Geometry check sheet. Reference: the model listing, model coordinates, mm. Face numbers are marked on the shaded views. Coordinates: 2 decimals unless noted, no trailing zeros. Loops run counter-clockwise (first coordinate to the right, second up) from the corner with the lowest first, then second, coordinate; pieces in that order, holes last.
from build123d import *

# Parameters (mm, degrees)
F0_W     = 266.7
F0_H     = 152.4
F0_R     = 19.05
F1_DEPTH = 50.8
F2_R     = 6.35


with BuildPart() as f1:
    # F0 (on Front) → F1 (new body)
    with BuildSketch(Plane.XZ):
        Rectangle(F0_W, F0_H)
        with Locations((-63.5, 0)):
            Circle(F0_R, mode=Mode.SUBTRACT)
        with BuildLine():
            ThreePointArc((-19.05, 0), (0, 19.05), (19.05, 0))
            ThreePointArc((19.05, 0), (0, -19.05), (-19.05, 0))
        make_face(mode=Mode.SUBTRACT)
        with BuildLine():
            ThreePointArc((82.55, 0), (63.5, -19.05), (44.45, 0))
            ThreePointArc((44.45, 0), (63.5, 19.05), (82.55, 0))
        make_face(mode=Mode.SUBTRACT)
    extrude(amount=F1_DEPTH)

    # F2
    f2_edges = [f1.edges().sort_by_distance(p)[0] for p in [
        (0, -50.8, 76.2),
        (-133.35, -50.8, 0),
        (0, -50.8, -76.2),
        (133.35, -50.8, 0),
    ]]
    fillet(f2_edges, radius=F2_R)


solid = f1.part
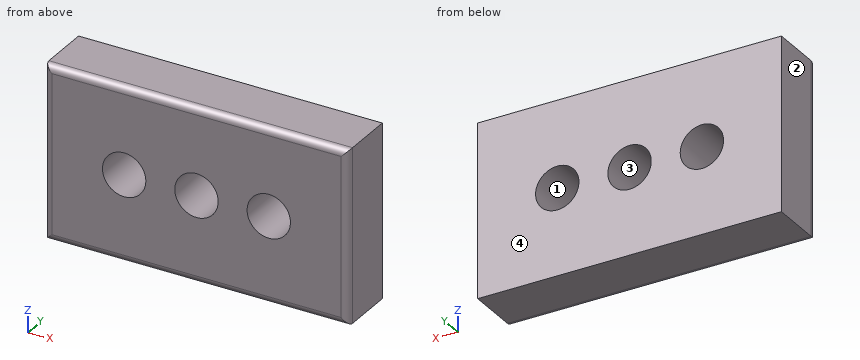
(1) Sectioned sample at D-D on x = -51. Record the cut outline in (y, z).
Findings:
outline: (-50.8, -69.85) arc R6.35 ccw to (-44.45, -76.2) - (0, -76.2) - (0, -14.38) - (-50.8, -14.38) - close; (-50.8, 14.38) - (0, 14.38) - (0, 76.2) - (-44.45, 76.2) arc R6.35 ccw to (-50.8, 69.85) - close
(2) Sectioned sample at A-A on z = 0. Record the cut outline in (x, y), and give its area (3 significant figures).
Findings:
outline: (-133.35, -44.45) arc R6.35 ccw to (-127, -50.8) - (-82.55, -50.8) - (-82.55, 0) - (-133.35, 0) - close; (-44.45, -50.8) - (-19.05, -50.8) - (-19.05, 0) - (-44.45, 0) - close; (19.05, -50.8) - (44.45, -50.8) - (44.45, 0) - (19.05, 0) - close; (82.55, -50.8) - (127, -50.8) arc R6.35 ccw to (133.35, -44.45) - (133.35, 0) - (82.55, 0) - close
area: 7,720 mm2
(3) Draft check along X on the marked faces 1, 2, 3 and 4. Enter one of: +X half, -X half, draft (parallel to the pull), parting line (faces both ways), or undercut.
Findings:
face 1: undercut
face 2: -X half
face 3: undercut
face 4: draft
(4) Sectioned sample at C-C on x = 63.5. Record the cut outline in (y, z), and give its area (3 significant figures).
Findings:
outline: (-50.8, -69.85) arc R6.35 ccw to (-44.45, -76.2) - (0, -76.2) - (0, -19.05) - (-50.8, -19.05) - close; (-50.8, 19.05) - (0, 19.05) - (0, 76.2) - (-44.45, 76.2) arc R6.35 ccw to (-50.8, 69.85) - close
area: 5,790 mm2
(5) Sectioned sample at B-B on y = -38. Record the cut outline in (x, z).
Findings:
outline: (-133.35, -76.2) - (133.35, -76.2) - (133.35, 76.2) - (-133.35, 76.2) - close; hole circle Ø38.1 at (-63.5, 0); hole circle Ø38.1 at (0, 0); hole circle Ø38.1 at (63.5, 0)
(6) Scan lines: L1, parallel to Z at x = 63.5, y = -40; L2, parallel to X at y = -29, z = -8.5; L3, parallel to X at y = -38, z = 11. Record each from-to range of solid material in increasing order.
Findings:
L1: z = -76.2 to -19.05, 19.05 to 76.2
L2: x = -133.35 to -80.55, -46.45 to -17.05, 17.05 to 46.45, 80.55 to 133.35
L3: x = -133.35 to -79.05, -47.95 to -15.55, 15.55 to 47.95, 79.05 to 133.35
